The listing builds one solid part. Answer for the finished solid, in the listing's coordinates (mm). A direction names the side the tool comes from. Round coordinates to 2 decimals unless told otherwise and drop trailing zeros. Write each loop counter-clockwise with the first axis right and the second up, starting at its lowest first coordinate (ties: lowest second). Pieces come first, ordered by that corner, then holes. Notation, with made-up numbers: M -18,-36.75 L 41,-36.75 A23 cw 41,-3.75 Z; hole C -16.75,55.25 d11. An arc over 180 degrees is marked long. One line per item, written item: value. Start each with the question number.
(1) Section A-A (z = 0.95) is taken. Determine the outline of the cut face in (x, y), plus the area to 3 significant figures.
(2) Section D-D (z = 1.5) is taken. Determine the outline of the cut face in (x, y).
(3) For a pull along X with two mould halves and no side action, classify faces 5 (the flat face through (0, -1, 0)), 6 (the flat face through (2.5, -2, 1)), 7 (the flat face through (0, -1, 2.8)) as released by +X, released by -X, zero draft, split by the parting line, or undercut.
(4) For faces 1 (the flat face through (0, 0, 1)), 2 (the flat face through (0, -4, 1.7)), 3 (the flat face through (0, -4, 1.2)), 4 (the flat face through (-2.5, -2, 1)), determine the directions among +Z, -Z, +X, -X, +Y, -Y from which every point of the face is accessible in a straight line to the end or side of a thin tool.
(5) Consider probe 1 along Y at (x, z) = (1.75, 0.7); probe 2 along Z at (x, y) = (0.25, -4.8); probe 3 along X at (y, z) = (-1.15, 0.3). Determine where each line is inside the solid, lowest interval first.
(6) Section C-C (y = -5.3) is taken. Determine the outline of the cut face in (x, z).
(7) Given P1, Ø1.5, axis at y = -2, z = 2, coming from the -X side; P2, Ø0.8, axis at x = -1, y = -1, coming from the +Z side; P3, Ø1, axis at x = -0.5, y = -4.5, coming from the -Z side, each flat-ended and moving along its own axis, determine where each tip first touches the part or whether it passes through.
(8) Section B-B (x = 0) is taken. Determine the outline of the cut face in (y, z).
```python
from build123d import *

# Parameters (mm, degrees)
BOX064_W     = 4
BOX064_H     = 0.6
BOX064_DEPTH = 0.2
BOX063_W     = 6.5
BOX063_H     = 0.6
BOX063_DEPTH = 3
BOX066_W     = 4
BOX066_H     = 3.5
BOX066_DEPTH = 0.5
BOX065_W     = 5
BOX065_H     = 2.5
BOX065_DEPTH = 2.8


with BuildPart() as cube037:
    # Box064 → Box064 (new body)
    with BuildSketch(Plane(origin=(-2, -0.6, 2.8), x_dir=(1, 0, 0), z_dir=(0, 0, 1))):
        with Locations((2, 0.3)):
            Rectangle(BOX064_W, BOX064_H)
    extrude(amount=BOX064_DEPTH)


with BuildPart() as cut015:
    # Box063 → Box063 (new body)
    with BuildSketch(Plane(origin=(-3.25, -0.6, 0), x_dir=(1, 0, 0), z_dir=(0, 0, 1))):
        with Locations((3.25, 0.3)):
            Rectangle(BOX063_W, BOX063_H)
    extrude(amount=BOX063_DEPTH)

    # Cut014: cut Cube037
    add(cube037.part, mode=Mode.SUBTRACT)


with BuildPart() as cube039:
    # Box066 → Box066 (new body)
    with BuildSketch(Plane(origin=(-2, -6, 1.2), x_dir=(1, 0, 0), z_dir=(0, 0, 1))):
        with Locations((2, 1.75)):
            Rectangle(BOX066_W, BOX066_H)
    extrude(amount=BOX066_DEPTH)


with BuildPart() as body008:
    # Box065 → Box065 (new body)
    with BuildSketch(Plane(origin=(-2.5, -2.5, 0), x_dir=(1, 0, 0), z_dir=(0, 0, 1))):
        with Locations((2.5, 1.25)):
            Rectangle(BOX065_W, BOX065_H)
    extrude(amount=BOX065_DEPTH)

    # Fusion048: union Cut015, Cube039
    add(cut015.part)
    add(cube039.part)


solid = body008.part
```
Recorded:
1. outline: M -3.25,-0.6 L -2.5,-0.6 L -2.5,-2.5 L 2.5,-2.5 L 2.5,-0.6 L 3.25,-0.6 L 3.25,0 L -3.25,0 Z
1. area: 13.4 mm2
2. outline: M -3.25,-0.6 L -2.5,-0.6 L -2.5,-2.5 L -2,-2.5 L -2,-6 L 2,-6 L 2,-2.5 L 2.5,-2.5 L 2.5,-0.6 L 3.25,-0.6 L 3.25,0 L -3.25,0 Z
3. face 5: zero draft
3. face 6: released by +X
3. face 7: undercut
4. face 1: +Z, -Z, +X, -X, +Y
4. face 2: +Z, +X, -X, -Y
4. face 3: -Z, +X, -X, -Y
4. face 4: +Z, -Z, -X, -Y
5. probe 1: y = -2.5 to 0
5. probe 2: z = 1.2 to 1.7
5. probe 3: x = -2.5 to 2.5
6. outline: M -2,1.2 L 2,1.2 L 2,1.7 L -2,1.7 Z
7. P1: stops at x = -2.5
7. P2: stops at z = 2.8
7. P3: stops at z = 1.2
8. outline: M -6,1.2 L -2.5,1.2 L -2.5,0 L 0,0 L 0,2.8 L -2.5,2.8 L -2.5,1.7 L -6,1.7 Z
